Can you work these out from the model? Positions are in its coordinate system, mm. A direction names the side the tool comes from. Give positions to 0.01 mm unless a question says otherwise; leave off trailing zeros. Order: outer loops, then holes, each group sorted by start corner. A loop starts at its lowest first (then second) coordinate and runs counter-clockwise, first axis right, second up. Notation, with made-up numbers: (59, -35) -> (92, -35) arc R21 cw to (92, -30) -> close; hole circle Ø6 at (0.25, -17). An arc over 180 degrees is marked (long way). Answer as a JSON object with one key per item and string values.
```python
from build123d import *

# Parameters (mm, degrees)
SKETCH1_R                               = 17.78
BOSS_EXTRUDE1_DEPTH                     = 7.62
SKETCH2_R                               = 10.795
BOSS_EXTRUDE2_DEPTH                     = 4.572
M2X0_4_TAPPED_HOLE1_D                   = 1.6
CBORE_FOR_M5_HEX_HEAD_BOLT1_D           = 18.288
CBORE_FOR_M5_HEX_HEAD_BOLT1_CBORE_D     = 19.304
CBORE_FOR_M5_HEX_HEAD_BOLT1_CBORE_DEPTH = 5.08


with BuildPart() as part:
    # Sketch1 → Boss-Extrude1 (new body)
    with BuildSketch(Plane(origin=(0, 0, 0), x_dir=(1, 0, 0), z_dir=(0, 1, 0))):
        Circle(SKETCH1_R)
    extrude(amount=BOSS_EXTRUDE1_DEPTH)

    # Sketch2 → Boss-Extrude2 (add)
    with BuildSketch(Plane(origin=(0, 7.62, 0), x_dir=(1, 0, 0), z_dir=(0, 1, 0))):
        Circle(SKETCH2_R)
    extrude(amount=BOSS_EXTRUDE2_DEPTH)

    # M2x0.4 Tapped Hole1 (through all)
    with Locations(Plane(origin=(0, 0, 0), x_dir=(-1, 0, 0), z_dir=(0, -1, 0))):
        with Locations((0, 15.875), (13.748153285, 7.9375), (13.748153285, -7.9375), (0, -15.875), (-13.748153285, -7.9375), (-13.748153285, 7.9375)):
            Hole(M2X0_4_TAPPED_HOLE1_D / 2)

    # CBORE for M5 Hex Head Bolt1 (through all)
    with Locations(Plane(origin=(0, 0, 0), x_dir=(-1, 0, 0), z_dir=(0, -1, 0))):
        with Locations((0, 0)):
            CounterBoreHole(CBORE_FOR_M5_HEX_HEAD_BOLT1_D / 2, CBORE_FOR_M5_HEX_HEAD_BOLT1_CBORE_D / 2, CBORE_FOR_M5_HEX_HEAD_BOLT1_CBORE_DEPTH)


solid = part.part
```
1. If we section it at A-A on x = 0: Please give me the cut outline in (y, z) (3 decimals).
Worked answers:
{"outline": "(0, -17.78) -> (7.62, -17.78) -> (7.62, -16.675) -> (0, -16.675) -> close; (0, -15.075) -> (7.62, -15.075) -> (7.62, -10.795) -> (12.192, -10.795) -> (12.192, -9.144) -> (5.08, -9.144) -> (5.08, -9.652) -> (0, -9.652) -> close; (0, 9.652) -> (5.08, 9.652) -> (5.08, 9.144) -> (12.192, 9.144) -> (12.192, 10.795) -> (7.62, 10.795) -> (7.62, 15.075) -> (0, 15.075) -> close; (0, 16.675) -> (7.62, 16.675) -> (7.62, 17.78) -> (0, 17.78) -> close"}
2. If we section it at B-B on z = 0: Please give me the cut outline in (x, y) (3 decimals).
Worked answers:
{"outline": "(-17.78, 0) -> (-9.652, 0) -> (-9.652, 5.08) -> (-9.144, 5.08) -> (-9.144, 12.192) -> (-10.795, 12.192) -> (-10.795, 7.62) -> (-17.78, 7.62) -> close; (9.144, 5.08) -> (9.652, 5.08) -> (9.652, 0) -> (17.78, 0) -> (17.78, 7.62) -> (10.795, 7.62) -> (10.795, 12.192) -> (9.144, 12.192) -> close"}
3. If we section it at D-D on x = -13.5: Please give me the cut outline in (y, z), then the cut area to 3 significant figures.
Worked answers:
{"outline": "(0, -11.57) -> (7.62, -11.57) -> (7.62, -8.7) -> (0, -8.7) -> close; (0, -7.18) -> (7.62, -7.18) -> (7.62, 7.18) -> (0, 7.18) -> close; (0, 8.7) -> (7.62, 8.7) -> (7.62, 11.57) -> (0, 11.57) -> close", "area": "153 mm²"}
4. For faces 1 (the face through (0.369, 3.863, 16.585)), 2 (the face through (7.66, 2.5, 5.87)), 3 (the face through (8, 7.62, 8)), which set-ups out of +Z, -Z, +X, -X, +Y, -Y let a thin tool reach every point of the face, with its end or its side?
Worked answers:
{"face 1": "+Y, -Y", "face 2": "-Y", "face 3": "+Y"}
5. Please list where these lines run through material, in increasing order: L1, parallel to Z at x = 0, y = 2.75 (3 decimals); L2, parallel to Z at x = 0, y = 9.5 (3 decimals); L3, parallel to Y at x = -9, z = -7.5.
Worked answers:
{"L1": "-17.78 to -16.675, -15.075 to -9.652, 9.652 to 15.075, 16.675 to 17.78", "L2": "-10.795 to -9.144, 9.144 to 10.795", "L3": "0 to 7.62"}
6. If we section it at C-C on y = 3.5: Please give me the cut outline in (x, z) (1 decimal).
Worked answers:
{"outline": "circle Ø35.6 at (0, 0); hole circle Ø1.6 at (-13.7, -7.9); hole circle Ø1.6 at (-13.7, 7.9); hole circle Ø19.3 at (0, 0); hole circle Ø1.6 at (0, -15.9); hole circle Ø1.6 at (0, 15.9); hole circle Ø1.6 at (13.7, -7.9); hole circle Ø1.6 at (13.7, 7.9)"}
7. Will these pins go through, and if not, where does the flat tip stop? pin 1 Ø1.5 at (x, z) = (4, -5.5) entering from -Y; pin 2 Ø1.8 at (x, z) = (0, -15.875) entering from +Y; pin 3 Ø1.5 at (y, z) = (4.5, -8.5) entering from +X; pin 4 Ø1.5 at (y, z) = (9.5, 9) entering from +X.
Worked answers:
{"pin 1": "through", "pin 2": "y = 7.62", "pin 3": "x = 16", "pin 4": "x = 6.96"}
8. If we mould it in two halves opening along X, with no side actions, what happens to faces 4 (the face through (-5, 5.08, 8)), 5 (the face through (8, 0, 8)), 6 (the face through (-7.956, 9.874, -7.296))? For each: +X half, -X half, draft (parallel to the pull), parting line (faces both ways), or undercut.
Worked answers:
{"face 4": "undercut", "face 5": "draft", "face 6": "parting line"}
